The model under review builds one solid part; all positions refer to its coordinate system, in mm. Face numbers are marked on the shaded views. A direction names the side the tool comes from. Coordinates: 2 decimals unless noted, no trailing zeros. Order: outer loops, then holes, each group sorted by start corner. A loop starts at its lowest first (then second) coordinate and runs counter-clockwise, first axis right, second up. Notation, with made-up numbers: (-9, -1.5) -> (31, -1.5) arc R12 ccw to (31, 21.5) -> close; hole circle Ø8 at (-32, -20.75). An arc over 180 degrees is marked (long way). Use CSV: the item, a comma, the result in double quotes. Start each with the question number.
```python
from build123d import *

# Parameters (mm, degrees)
BOSS_EXTRUDE1_DEPTH         = 101.6
FILLET1_R                   = 6.35
FILLET2_R                   = 6.35
F_3_8_16_TAPPED_HOLE3_D     = 7.9375
F_3_8_16_TAPPED_HOLE3_DEPTH = 16.002
F_3_8_16_TAPPED_HOLE3_TIP   = 2.384665582
F_3_8_16_TAPPED_HOLE4_D     = 7.9375
BOSS_EXTRUDE2_DEPTH         = 31.75


with BuildPart() as part:
    # Sketch1 → Boss-Extrude1 (new body)
    with BuildSketch(Plane.XY):
        Polygon((-58.674, 0), (-58.674, 6.35), (-6.35, 6.35), (-6.35, 0), (0, 0), (0, 31.75), (-65.024, 31.75), (-65.024, 0), align=None)
    extrude(amount=BOSS_EXTRUDE1_DEPTH)

    # Fillet1
    fillet1_edges = [part.edges().sort_by_distance(p)[0] for p in [
        (-6.35, 6.35, 50.8),
    ]]
    fillet(fillet1_edges, radius=FILLET1_R - 0.0001)  # a hair under: the kernel refuses the full size

    # Fillet2
    fillet2_edges = [part.edges().sort_by_distance(p)[0] for p in [
        (-58.674, 6.35, 50.8),
    ]]
    fillet(fillet2_edges, radius=FILLET2_R - 0.0001)  # a hair under: the kernel refuses the full size

    # 3/8-16 Tapped Hole3
    with Locations(Plane(origin=(0, 0, 0), x_dir=(-1, 0, 0), z_dir=(0, 0, -1))):
        with Locations((31.75, 22.352)):
            Hole(F_3_8_16_TAPPED_HOLE3_D / 2, depth=F_3_8_16_TAPPED_HOLE3_DEPTH)
            with Locations((0, 0, -(F_3_8_16_TAPPED_HOLE3_DEPTH + F_3_8_16_TAPPED_HOLE3_TIP / 2))):  # 118° drill point
                Cone(0, F_3_8_16_TAPPED_HOLE3_D / 2, F_3_8_16_TAPPED_HOLE3_TIP, mode=Mode.SUBTRACT)

    # 3/8-16 Tapped Hole4 (through all)
    with Locations(Plane(origin=(0, 0, 0), x_dir=(0, 0, -1), z_dir=(1, 0, 0))):
        with Locations((-50.8, 16.002)):
            Hole(F_3_8_16_TAPPED_HOLE4_D / 2)

    # Sketch13 → Boss-Extrude2 (add)
    with BuildSketch(Plane.XY):
        Polygon((-14.224, 31.75), (-14.224, 38.1), (-7.112, 38.1), (-7.112, 69.85), (-13.462, 69.85), (-29.21, 54.102), (-29.21, 47.752), (-35.814, 47.752), (-35.814, 54.102), (-51.562, 69.85), (-57.912, 69.85), (-57.912, 38.1), (-50.8, 38.1), (-50.8, 31.75), align=None)
    boss_extrude2 = extrude(amount=BOSS_EXTRUDE2_DEPTH)

    # Mirror1: Boss-Extrude2 across plane
    add(boss_extrude2.mirror(Plane.XY.offset(50.8)))


solid = part.part
```
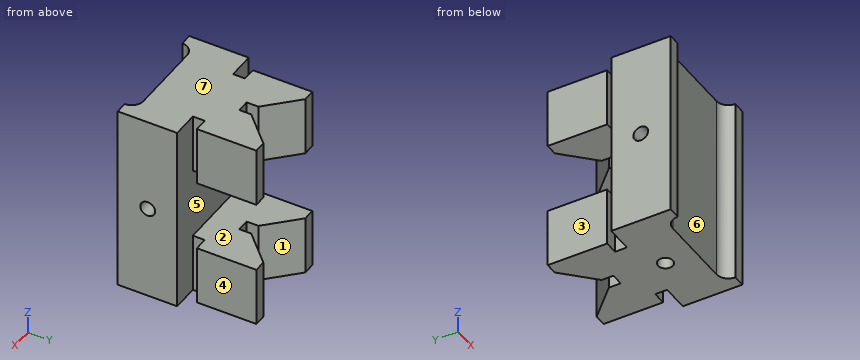
Q1. For the marked faces 1, 2, 3 and 4, list the 3-axis set-ups (+Z, -Z, +X, -X, +Y, -Y) from which the entire face can be reached by the end or side of a thin tool; tool diameter is ignored.
Q2. Draft analysis for pull direction Y (two halves, no side actions). For the marked faces 5, 6 and 7, state which applies: +Y half, -Y half, draft (parallel to the pull), parting line (faces both ways), or undercut.
Q3. Add section D-D, the plane y = 57.5. State the section outline as (x, z) points.
Q4. Clearance check with flat-ended pins moving along their axes: pin 1 Ø9.5 at (y, z) = (59.5, 88) entering from +X; pin 2 Ø7.5 at (x, z) = (-32.5, 10.5) entering from +Y; pin 3 Ø5 at (y, z) = (34.5, 79.5) entering from +X. State where each tip first meets the part, or that it passes through.
Q5. Add section B-B, the plane x = -60.5. State the section outline as (y, z) points, then the cut area to 3 significant figures.
Q6. To check wall thickness, follow probe 1 along Y at (x, z) = (-19, 50.8); probe 2 along Y at (x, z) = (-31.75, 9.25); probe 3 along Z at (x, y) = (-19.5, 32.5). State the ranges of each line that lie inside material, in increasing order.
Q7. Add section C-C, the plane y = 46. State the section outline as (x, z) points.
Answer block:
1,face 1,"+Z, -Z, +Y"
1,face 2,"+X, -X, +Y"
1,face 3,"+Z, -Z, -X, +Y"
1,face 4,"+Z, -Z, +X, +Y"
2,face 5,"undercut"
2,face 6,"-Y half"
2,face 7,"draft"
3,outline,"(-57.91, 0) -> (-39.21, 0) -> (-39.21, 31.75) -> (-57.91, 31.75) -> close; (-57.91, 69.85) -> (-39.21, 69.85) -> (-39.21, 101.6) -> (-57.91, 101.6) -> close; (-25.81, 0) -> (-7.11, 0) -> (-7.11, 31.75) -> (-25.81, 31.75) -> close; (-25.81, 69.85) -> (-7.11, 69.85) -> (-7.11, 101.6) -> (-25.81, 101.6) -> close"
4,pin 1,"stops at x = -7.11"
4,pin 2,"stops at y = 54.56"
4,pin 3,"stops at x = -14.22"
5,outline,"(0, 0) -> (31.75, 0) -> (31.75, 101.6) -> (0, 101.6) -> close; hole circle Ø7.94 at (16, 50.8)"
5,area,"3,180 mm²"
6,probe 1,"y = 6.35 to 12.03, 19.97 to 31.75"
6,probe 2,"y = 6.35 to 18.38, 26.32 to 47.75"
6,probe 3,"z = 0 to 31.75, 69.85 to 101.6"
7,outline,"(-57.91, 0) -> (-7.11, 0) -> (-7.11, 31.75) -> (-57.91, 31.75) -> close; (-57.91, 69.85) -> (-7.11, 69.85) -> (-7.11, 101.6) -> (-57.91, 101.6) -> close"
